```python
from build123d import *

# Parameters (mm, degrees)
STOCK_NEW_TRACKER_1_START = 60
STOCK_NEW_TRACKER_1_DEPTH = 8
SKETCH1_R                 = 9.25
CUT_EXTRUDE1_DEPTH        = 1
SKETCH2_R                 = 8.05
CUT_EXTRUDE2_DEPTH        = 143.502485249
M4X0_7_TAPPED_HOLE1_D     = 3.3
M4X0_7_TAPPED_HOLE1_DEPTH = 35
M4X0_7_TAPPED_HOLE1_TIP   = 0.991420021


# Read off the part's stored shape, not the designer's step: Stock-New_Tracker-1
with BuildPart() as part:
    # Stock-New_Tracker-1 outline → Stock-New_Tracker-1 (new body)
    with BuildSketch(Plane.YZ.offset(STOCK_NEW_TRACKER_1_START)):
        with BuildLine():
            Line((10, 40), (10, -40))
            Line((10, -40), (96.116983094, -40))
            ThreePointArc((96.116983094, -40), (124.570453884, -28.312888011), (136.594137144, 0))
            ThreePointArc((136.594137144, 0), (124.570453884, 28.312888011), (96.116983094, 40))
            Line((96.116983094, 40), (10, 40))
        make_face()
    extrude(amount=STOCK_NEW_TRACKER_1_DEPTH)

    # Sketch1 → Cut-Extrude1 (cut)
    with BuildSketch(Plane(origin=(68, 0, 0), x_dir=(0, 0, -1), z_dir=(1, 0, 0))):
        with Locations((-0.48, 96.116983094)):
            Circle(SKETCH1_R)
    extrude(amount=-CUT_EXTRUDE1_DEPTH, mode=Mode.SUBTRACT)

    # Sketch2 → Cut-Extrude2 (cut, through all)
    with BuildSketch(Plane(origin=(67, 0, 0), x_dir=(0, 0, -1), z_dir=(1, 0, 0))):
        with Locations((-0.48, 96.116983094)):
            Circle(SKETCH2_R)
    extrude(amount=-CUT_EXTRUDE2_DEPTH, mode=Mode.SUBTRACT)

    # M4x0.7 Tapped Hole1
    with Locations(Plane(origin=(0, 10, 0), x_dir=(-1, 0, 0), z_dir=(0, -1, 0))):
        with Locations((-64, -30), (-64, 0), (-64, 30)):
            Hole(M4X0_7_TAPPED_HOLE1_D / 2, depth=M4X0_7_TAPPED_HOLE1_DEPTH)
            with Locations((0, 0, -(M4X0_7_TAPPED_HOLE1_DEPTH + M4X0_7_TAPPED_HOLE1_TIP / 2))):  # 118° drill point
                Cone(0, M4X0_7_TAPPED_HOLE1_D / 2, M4X0_7_TAPPED_HOLE1_TIP, mode=Mode.SUBTRACT)


solid = part.part
```
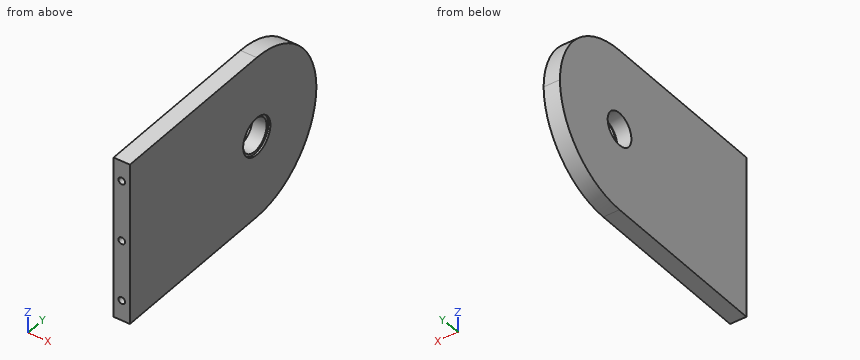
Geometry check sheet. Reference: the model listing, model coordinates, mm. Coordinates: 2 decimals unless noted, no trailing zeros. Order: outer loops, then holes, each group sorted by start corner. A loop starts at its lowest first (then second) coordinate and runs counter-clockwise, first axis right, second up. Notation, with made-up numbers: (73.25, 36.5) - (100.25, 36.5) arc R22 ccw to (100.25, 71.5) - close; hole circle Ø6 at (19, 8). An arc over 180 degrees is marked (long way). Answer in a Markdown table with one row per item. Add a question column.
1. Section check C-C (y = 112). Enter the section's corners in (x, z).
2. Material ranges on L1, parallel to Z at x = 64, y = 21; L2, parallel to X at y = 20, z = 30; L3, parallel to Y at x = 67.2, z = 0.48, recorded low to high. Write a range as [from, to].
3. Section check A-A (y = 22). Enter the section's corners in (x, z), plus the area to 3 significant figures.
4. Gauge pin test, flat ends, axial feed: pin 1 Ø2 at (x, z) = (64, 30) entering from +Y; pin 2 Ø2 at (x, z) = (64, 0) entering from -Y. Record the tip position at first contact, or that the pin passes through.
5. Section check B-B (z = -22). Enter the section's corners in (x, y).
Data:
| question | item | result |
|---|---|---|
| 1 | outline | (60, -36.75) - (68, -36.75) - (68, 36.75) - (60, 36.75) - close |
| 2 | L1 | z = [-40, -31.65], [-28.35, -1.65], [1.65, 28.35], [31.65, 40] |
| 2 | L2 | x = [60, 62.35], [65.65, 68] |
| 2 | L3 | y = [10, 86.87], [105.37, 136.59] |
| 3 | outline | (60, -40) - (68, -40) - (68, 40) - (60, 40) - close; hole circle Ø3.3 at (64, -30); hole circle Ø3.3 at (64, 0); hole circle Ø3.3 at (64, 30) |
| 3 | area | 614 mm² |
| 4 | pin 1 | stops at y = 123.86 |
| 4 | pin 2 | stops at y = 45.39 |
| 5 | outline | (60, 10) - (68, 10) - (68, 129.78) - (60, 129.78) - close |
